from build123d import *

# Parameters (mm, degrees)
F0_W        = 50
F0_H        = 18
F0_R        = 6.5
F1_DEPTH    = 50
F2_R        = 6.5
F3_DEPTH    = 3
F4_T1_DEPTH = 143
F5_R        = 5.25
F6_DEPTH    = 25


# Not quite as in the source:
# - a fillet or chamfer that OpenCascade refuses, or shapes differently, is made with other operations: its cross-section is extruded or revolved along the edge and cut away or added


with BuildPart() as f1:
    # F0 (on Front) → F1 (new body)
    with BuildSketch(Plane.XZ):
        Rectangle(F0_W, F0_H)
        Circle(F0_R, mode=Mode.SUBTRACT)
        Circle(F0_R)
    extrude(amount=F1_DEPTH)

    # F2 (on Front) → F3 (cut)
    with BuildSketch(Plane.XZ):
        Circle(F2_R)
    extrude(amount=F3_DEPTH, mode=Mode.SUBTRACT)

    # F4: fillet of radius 25 on 4 edges, made by hand

    # F4_s2 → F4_t1 (cut)
    with BuildSketch(Plane.XY.offset(-71.5)):
        with BuildLine():
            ThreePointArc((-25, -25), (-17.6776695297, -7.3223304703), (0, 0))
            Line((0, 0), (-25, 0))
            Line((-25, 0), (-25, -25))
        make_face()
        with BuildLine():
            ThreePointArc((25, -25), (17.6776695297, -7.3223304703), (0, 0))
            Line((0, 0), (25, 0))
            Line((25, 0), (25, -25))
        make_face()
        with BuildLine():
            ThreePointArc((25, -25), (17.6776695297, -42.6776695297), (0, -50))
            Line((0, -50), (25, -50))
            Line((25, -50), (25, -25))
        make_face()
        with BuildLine():
            ThreePointArc((-25, -25), (-17.6776695297, -42.6776695297), (0, -50))
            Line((0, -50), (-25, -50))
            Line((-25, -50), (-25, -25))
        make_face()
    extrude(amount=F4_T1_DEPTH, mode=Mode.SUBTRACT)

    # F5 (on face) → F6 (cut)
    with BuildSketch(Plane.XY.offset(9)):
        with Locations((0, -25)):
            Circle(F5_R)
    extrude(amount=-F6_DEPTH, mode=Mode.SUBTRACT)


solid = f1.part
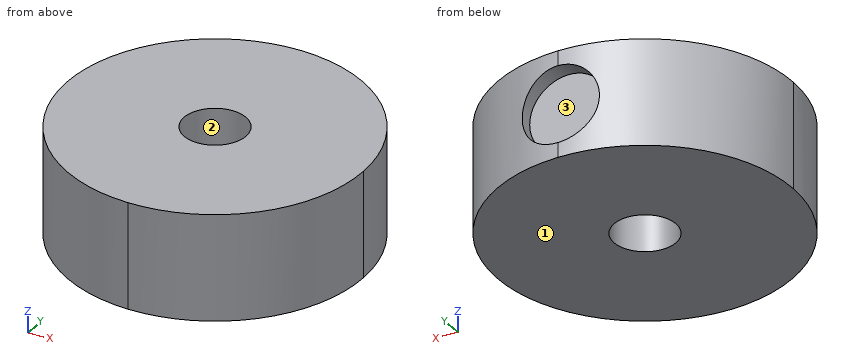
For this review, take the finished solid that the model builds, in its own axes (mm). Face numbers are marked on the shaded views. Coordinates: 2 decimals unless noted, no trailing zeros. Loops run counter-clockwise (first coordinate to the right, second up) from the corner with the lowest first, then second, coordinate; pieces in that order, holes last. Notation, with made-up numbers: (16.25, 12.5) - (68.25, 12.5) arc R26 ccw to (68.25, 44.5) - close; hole circle Ø6 at (59.25, -6.75). An arc over 180 degrees is marked (long way). Use a Markdown table: item, result. Add a question column.
Item 1: Insertion check: pin 1 Ø1 at (y, z) = (-22.5, 6.5) entering from +X; pin 2 Ø3 at (x, z) = (-7.5, 1) entering from -Y; pin 3 Ø10.5 at (x, z) = (0, 0) entering from +Y; pin 4 Ø9.5 at (x, y) = (0, -25) entering from +Z. Each pin has a flat end and moves straight along its axis. Give the tip position at first contact, or say it passes through.
Item 2: For line 1 (Y direction, x = 0, z = -1.75); line 2 (Y direction, x = 3.5, z = 5.75); line 3 (X direction, y = -26, z = 2.5), list the stretches that pass through material, from the lowest coordinate up.
Item 3: We need section B-B (x = 17). Give the boundary of the cut face in (y, z), and give its area (3 significant figures).
Item 4: We need section A-A (z = 0.75). Give the boundary of the cut face in (x, y).
Item 5: We need section C-C (y = -6.5). Give the boundary of the cut face in (x, z), and give its area (3 significant figures).
Item 6: Mouldability with a two-part tool opening along Y and no side actions: class the marked faces 1, 2 and 3 as pulls with the +Y half, pulls with the -Y half, needs draft (parallel to the pull), parting line crosses it, or undercut.
Results list:
| question | item | result |
|---|---|---|
| 1 | pin 1 | stops at x = 24.92 |
| 1 | pin 2 | stops at y = -49.27 |
| 1 | pin 3 | stops at y = -3 |
| 1 | pin 4 | passes through |
| 2 | line 1 | y = -50 to -30.25, -19.75 to -3 |
| 2 | line 2 | y = -49.75 to -28.91, -21.09 to -0.25 |
| 2 | line 3 | x = -24.98 to -5.15, 5.15 to 24.98 |
| 3 | outline | (-43.33, -9) - (-6.67, -9) - (-6.67, 9) - (-43.33, 9) - close |
| 3 | area | 660 mm^2 |
| 4 | outline | (-6.46, -3) - (-6.46, -0.85) arc R25 ccw (long way) to (6.46, -0.85) - (6.46, -3) - close; hole circle Ø10.5 at (0, -25) |
| 5 | outline | (-16.82, -9) - (16.82, -9) - (16.82, 9) - (-16.82, 9) - close |
| 5 | area | 605 mm^2 |
| 6 | face 1 | needs draft |
| 6 | face 2 | undercut |
| 6 | face 3 | pulls with the +Y half |
